Input: part model. Units: mm. Frame: model coordinates. Round coordinates to 2 decimals unless told otherwise and drop trailing zeros. Order: outer loops, then holes, each group sorted by start corner. A loop starts at its lowest first (then second) coordinate and runs counter-clockwise, first axis right, second up.
Item 1: Cut plane A-A on x = 0. Output: boundary loops of the cut face in (y, z), then the cut area to 3 significant figures.
Item 2: Cut plane B-B on z = -56.5. Output: boundary loops of the cut face in (x, y).
Item 3: Line query: L1, parallel to Z at x = 66.5, y = 2; L2, parallel to X at y = 1.75, z = 57; L3, parallel to X at y = 5.5, z = 0. Output: solid intervals per line, ascending.
Item 4: Cut plane D-D on z = 0. Output: boundary loops of the cut face in (x, y), then the cut area to 3 significant figures.
Item 5: Cut plane C-C on y = 5. Output: boundary loops of the cut face in (x, z).
```python
from build123d import *

# Parameters (mm, degrees)
SKETCH1_W           = 177.8
SKETCH1_H           = 152.4
BOSS_EXTRUDE1_DEPTH = 7.62
SKETCH2_R           = 12.7
CUT_EXTRUDE1_DEPTH  = 7.62
SKETCH3_W           = 12.7
SKETCH3_H           = 12.7
CUT_EXTRUDE2_DEPTH  = 118.335904139


with BuildPart() as part:
    # Sketch1 → Boss-Extrude1 (new body)
    with BuildSketch(Plane(origin=(0, 0, 0), x_dir=(1, 0, 0), z_dir=(0, 1, 0))):
        Rectangle(SKETCH1_W, SKETCH1_H)
    extrude(amount=BOSS_EXTRUDE1_DEPTH)

    # Sketch2 → Cut-Extrude1 (cut)
    with BuildSketch(Plane(origin=(0, 7.62, 0), x_dir=(1, 0, 0), z_dir=(0, 1, 0))):
        with Locations(Location((0, 0, 0), (0, 0, 270))):
            Circle(SKETCH2_R)
    extrude(amount=-CUT_EXTRUDE1_DEPTH, mode=Mode.SUBTRACT)

    # Sketch3 → Cut-Extrude2 (cut, through all)
    with BuildSketch(Plane(origin=(0, 7.62, 0), x_dir=(1, 0, 0), z_dir=(0, 1, 0))):
        with Locations((-69.85, -57.15)):
            Rectangle(SKETCH3_W, SKETCH3_H)
        with Locations((69.85, -57.15)):
            Rectangle(SKETCH3_W, SKETCH3_H)
        with Locations((-69.85, 57.15)):
            Rectangle(SKETCH3_W, SKETCH3_H)
        with Locations((69.85, 57.15)):
            Rectangle(SKETCH3_W, SKETCH3_H)
    extrude(amount=-CUT_EXTRUDE2_DEPTH, mode=Mode.SUBTRACT)


solid = part.part
```
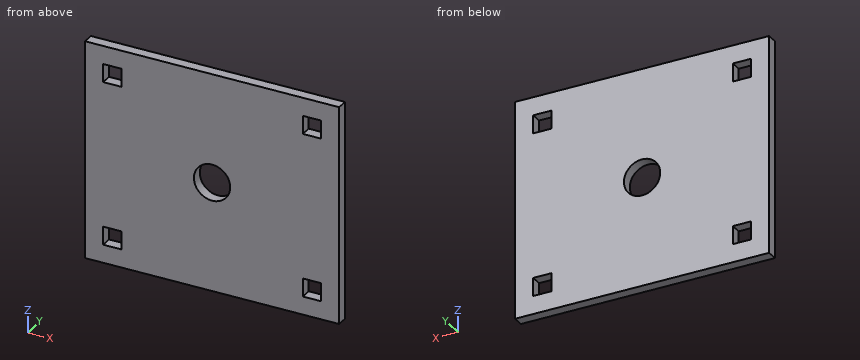
From the geometry:
1. outline: (0, -76.2) - (7.62, -76.2) - (7.62, -12.7) - (0, -12.7) - close; (0, 12.7) - (7.62, 12.7) - (7.62, 76.2) - (0, 76.2) - close
1. area: 968 mm2
2. outline: (-88.9, 0) - (-76.2, 0) - (-76.2, 7.62) - (-88.9, 7.62) - close; (-63.5, 0) - (63.5, 0) - (63.5, 7.62) - (-63.5, 7.62) - close; (76.2, 0) - (88.9, 0) - (88.9, 7.62) - (76.2, 7.62) - close
3. L1: z = -76.2 to -63.5, -50.8 to 50.8, 63.5 to 76.2
3. L2: x = -88.9 to -76.2, -63.5 to 63.5, 76.2 to 88.9
3. L3: x = -88.9 to -12.7, 12.7 to 88.9
4. outline: (-88.9, 0) - (-12.7, 0) - (-12.7, 7.62) - (-88.9, 7.62) - close; (12.7, 0) - (88.9, 0) - (88.9, 7.62) - (12.7, 7.62) - close
4. area: 1,160 mm2
5. outline: (-88.9, -76.2) - (88.9, -76.2) - (88.9, 76.2) - (-88.9, 76.2) - close; hole (-76.2, -63.5) - (-63.5, -63.5) - (-63.5, -50.8) - (-76.2, -50.8) - close; hole (-76.2, 50.8) - (-63.5, 50.8) - (-63.5, 63.5) - (-76.2, 63.5) - close; hole circle Ø25.4 at (0, 0); hole (63.5, -63.5) - (76.2, -63.5) - (76.2, -50.8) - (63.5, -50.8) - close; hole (63.5, 50.8) - (76.2, 50.8) - (76.2, 63.5) - (63.5, 63.5) - close
